Geometry: see drawing. Coordinates: mm, zero at the bounding-box minimum. Round coordinates to 2 decimals unless told otherwise and drop trailing zeros. Write each loop counter-clockwise with the first axis right and the second up, starting at its lowest first coordinate (ties: lowest second). Pieces come first, ordered by that corner, then holes. Notation, with made-up numbers: M 85.5,-12.5 L 128.5,-12.5 A30 cw 128.5,17.5 Z; hole C 80,-11 d3. An arc over 180 degrees is marked long. Use a Markdown table: item, result.
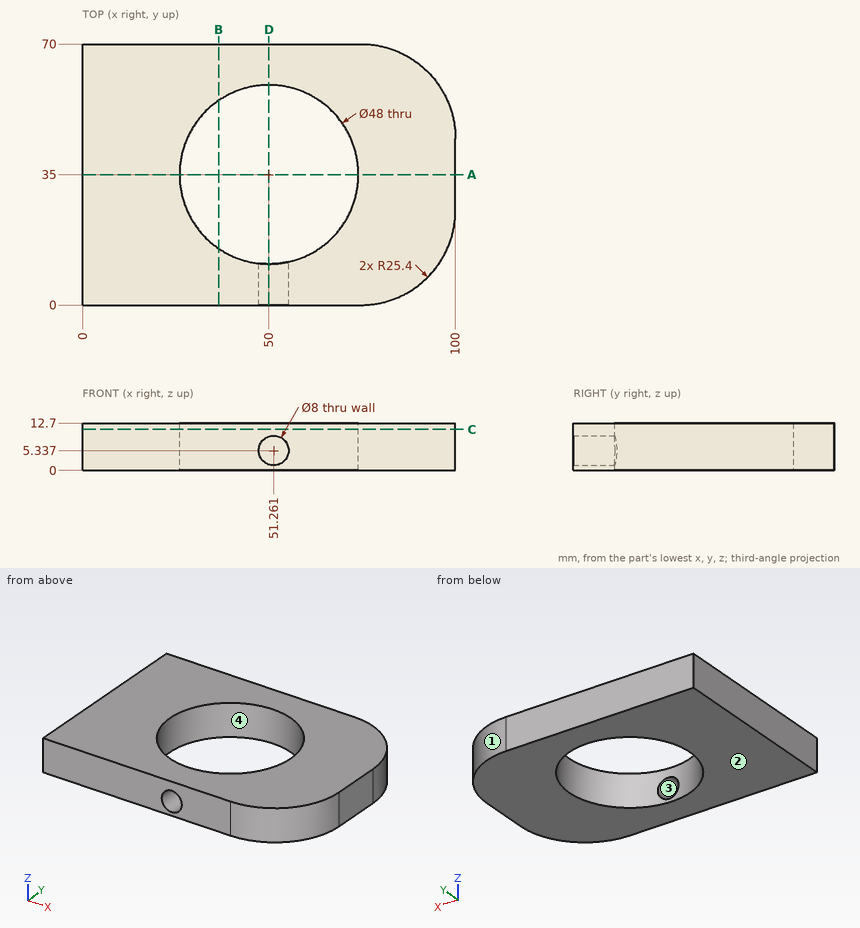
Q1. Section C-C on z = 11. Return loops of the section in (x, y), plus the area to 3 significant figures.
Results are:
| item | result |
|---|---|
| outline | M 0,0 L 74.6,0 A25.4 ccw 100,25.4 L 100,44.6 A25.4 ccw 74.6,70 L 0,70 Z; hole C 50,35 d48 |
| area | 4,910 mm^2 |
Q2. First-contact query: pin 1 Ø7 at (x, z) = (51.26, 5.34) entering from -Y; pin 2 Ø1.5 at (y, z) = (11.5, 10) entering from +X. Flat tips, straight axial feed; report the tip coordinate or a pass-through.
Results are:
| item | result |
|---|---|
| pin 1 | y = 58.52 |
| pin 2 | x = 96.33 |
Q3. Section A-A on y = 35. Return loops of the section in (x, z), plus the area to 3 significant figures.
Results are:
| item | result |
|---|---|
| outline | M 0,0 L 26,0 L 26,12.7 L 0,12.7 Z; M 74,0 L 100,0 L 100,12.7 L 74,12.7 Z |
| area | 660 mm^2 |
Q4. Line query: L1, parallel to Y at x = 28, z = 7.5 (1 decimal); L2, parallel to Y at x = 50.5, z = 9 (1 decimal); L3, parallel to Y at x = 70.5, z = 11.5. Output: solid intervals per line, ascending.
Results are:
| item | result |
|---|---|
| L1 | 0 to 25.4, 44.6 to 70 |
| L2 | 59 to 70 |
| L3 | 0 to 22.52, 47.48 to 70 |
Q5. Section B-B on x = 36.5. Return loops of the section in (y, z), plus the area to 3 significant figures.
Results are:
| item | result |
|---|---|
| outline | M 0,0 L 15.16,0 L 15.16,12.7 L 0,12.7 Z; M 54.84,0 L 70,0 L 70,12.7 L 54.84,12.7 Z |
| area | 385 mm^2 |
Q6. Section D-D on x = 50. Return loops of the section in (y, z).
Results are:
| item | result |
|---|---|
| outline | M 0,0 L 11,0 L 11,1.54 L 0,1.54 Z; M 0,9.13 L 11,9.13 L 11,12.7 L 0,12.7 Z; M 59,0 L 70,0 L 70,12.7 L 59,12.7 Z |
Q7. Mould query, pull axis X, two halves, no side actions, for the marked faces 1, 2, 3 and 4. Classes: +X half, -X half, draft (parallel to the pull), parting line (faces both ways), or undercut.
Results are:
| item | result |
|---|---|
| face 1 | +X half |
| face 2 | draft |
| face 3 | undercut |
| face 4 | undercut |
